Read the model definition and answer for the solid it produces. Units are mm, in the model's axes. Face numbers are marked on the shaded views. A direction names the side the tool comes from. Coordinates: 2 decimals unless noted, no trailing zeros. Write each loop counter-clockwise with the first axis right and the second up, starting at its lowest first coordinate (ties: lowest second). Pieces come first, ordered by that corner, then holes. Notation, with made-up numbers: (42.5, 87) -> (64.5, 87) arc R8 cw to (64.5, 93) -> close; hole circle Ø4 at (-22.75, 32.5). An arc over 180 degrees is marked (long way). Answer as a JSON object with one key per item and string values. Group by question number.
(1) Straight lines are drawn through the part: L1, parallel to Y at x = 2.25, z = 0; L2, parallel to X at y = -5.5, z = -2.5; L3, parallel to X at y = 5, z = 1.25. For each, find the intervals that lie inside material, in ascending order.
(2) Find section D-D (x = 22.5). Give the vertices of the cut face in (y, z), then the cut area to 3 significant figures.
(3) For a pull along Y with two mould halves and no side action, classify the marked faces 3, 4 and 5 as +Y half, -Y half, draft (parallel to the pull), parting line (faces both ways), or undercut.
(4) Find section B-B (x = 14.5). Give the vertices of the cut face in (y, z).
(5) Flat-ended cylindrical pins translate along their axes: P1, Ø0.6, axis at x = 25.5, z = -6.5, coming from the +Y side; P2, Ø7, axis at y = 3.5, z = 4.5, coming from the +X side; P3, Ø6, axis at y = 0, z = 0, coming from the -X side. Find the tip coordinate at first contact, or state that the pin passes through.
(6) Find section C-C (z = -6.25). Give the vertices of the cut face in (x, y).
(7) Find section A-A (z = 0). Give the vertices of the cut face in (x, y).
(8) Which of the six approach directions +Z, -Z, +X, -X, +Y, -Y give full straight-line access (tool end or side, diameter ignored) to the marked faces 1 and 2?
from build123d import *

# Parameters (mm, degrees)
SKETCH1_W           = 28.5
SKETCH1_H           = 15
SKETCH1_R           = 4.25
BOSS_EXTRUDE1_DEPTH = 6.2
SKETCH2_W           = 5
SKETCH2_H           = 15
BOSS_EXTRUDE2_DEPTH = 15
SKETCH3_W           = 5
SKETCH3_H           = 15
BOSS_EXTRUDE3_DEPTH = 5
CUT_EXTRUDE2_START  = 2
CUT_EXTRUDE2_DEPTH  = 1
CUT_EXTRUDE3_START  = 3
CUT_EXTRUDE3_DEPTH  = 2
FILLET1_R           = 3


with BuildPart() as part:
    # Sketch1 → Boss-Extrude1 (new body)
    with BuildSketch(Plane(origin=(0, 0, 0), x_dir=(0, 0, -1), z_dir=(1, 0, 0))):
        Rectangle(SKETCH1_W, SKETCH1_H)
        with Locations(Location((0, 0, 0), (0, 0, 180))):
            Circle(SKETCH1_R, mode=Mode.SUBTRACT)
    extrude(amount=BOSS_EXTRUDE1_DEPTH)

    # Sketch2 → Boss-Extrude2 (add)
    with BuildSketch(Plane(origin=(6.2, 0, 0), x_dir=(0, 0, -1), z_dir=(1, 0, 0))):
        with Locations((-11.75, 0)):
            Rectangle(SKETCH2_W, SKETCH2_H)
        with Locations((11.75, 0)):
            Rectangle(SKETCH2_W, SKETCH2_H)
    extrude(amount=BOSS_EXTRUDE2_DEPTH)

    # Sketch3 → Boss-Extrude3 (add)
    with BuildSketch(Plane(origin=(21.2, 0, 0), x_dir=(0, 0, -1), z_dir=(1, 0, 0))):
        with Locations((-11.75, 0)):
            Rectangle(SKETCH3_W, SKETCH3_H)
        with BuildLine():
            Line((8.525, -0.9), (8.525, 7.5))
            Line((8.525, 7.5), (-8.525, 7.5))
            Line((-8.525, 7.5), (-8.525, -0.9))
            Line((-8.525, -0.9), (-3.64039833, -0.9))
            ThreePointArc((-3.64039833, -0.9), (-0.453324532, 3.72249874), (3.75, 0))
            ThreePointArc((3.75, 0), (3.72249874, -0.453324532), (3.64039833, -0.9))
            Line((3.64039833, -0.9), (8.525, -0.9))
        make_face()
        with BuildLine():
            Line((-9.25, -7.5), (14.25, -7.5))
            Line((14.25, -7.5), (14.25, 7.5))
            Line((14.25, 7.5), (9.125, 7.5))
            Line((9.125, 7.5), (9.125, -1.5))
            Line((9.125, -1.5), (3.436931771, -1.5))
            ThreePointArc((3.436931771, -1.5), (0, -3.75), (-3.436931771, -1.5))
            Line((-3.436931771, -1.5), (-9.125, -1.5))
            Line((-9.125, -1.5), (-9.125, 7.5))
            Line((-9.125, 7.5), (-9.25, 7.5))
            Line((-9.25, 7.5), (-9.25, -7.5))
        make_face()
        with BuildLine():
            Line((-8.525, 7.5), (-9.125, 7.5))
            Line((-9.125, 7.5), (-9.125, -1.5))
            Line((-9.125, -1.5), (-3.436931771, -1.5))
            ThreePointArc((-3.436931771, -1.5), (-3.551358943, -1.204304638), (-3.64039833, -0.9))
            Line((-3.64039833, -0.9), (-8.525, -0.9))
            Line((-8.525, -0.9), (-8.525, 7.5))
        make_face()
        with BuildLine():
            Line((9.125, -1.5), (9.125, 7.5))
            Line((9.125, 7.5), (8.525, 7.5))
            Line((8.525, 7.5), (8.525, -0.9))
            Line((8.525, -0.9), (3.64039833, -0.9))
            ThreePointArc((3.64039833, -0.9), (3.551358943, -1.204304638), (3.436931771, -1.5))
            Line((3.436931771, -1.5), (9.125, -1.5))
        make_face()
    extrude(amount=BOSS_EXTRUDE3_DEPTH)

    # Sketch3<6> → Cut-Extrude2 (cut)
    with BuildSketch(Plane(origin=(21.2, 0, 0), x_dir=(0, 0, -1), z_dir=(1, 0, 0)).offset(CUT_EXTRUDE2_START)):
        with BuildLine():
            Line((8.525, -0.9), (8.525, 7.5))
            Line((8.525, 7.5), (-8.525, 7.5))
            Line((-8.525, 7.5), (-8.525, -0.9))
            Line((-8.525, -0.9), (-3.64039833, -0.9))
            ThreePointArc((-3.64039833, -0.9), (-0.453324532, 3.72249874), (3.75, 0))
            ThreePointArc((3.75, 0), (3.72249874, -0.453324532), (3.64039833, -0.9))
            Line((3.64039833, -0.9), (8.525, -0.9))
        make_face()
        with BuildLine():
            Line((-8.525, 7.5), (-9.125, 7.5))
            Line((-9.125, 7.5), (-9.125, -1.5))
            Line((-9.125, -1.5), (-3.436931771, -1.5))
            ThreePointArc((-3.436931771, -1.5), (-3.551358943, -1.204304638), (-3.64039833, -0.9))
            Line((-3.64039833, -0.9), (-8.525, -0.9))
            Line((-8.525, -0.9), (-8.525, 7.5))
        make_face()
        with BuildLine():
            Line((9.125, -1.5), (9.125, 7.5))
            Line((9.125, 7.5), (8.525, 7.5))
            Line((8.525, 7.5), (8.525, -0.9))
            Line((8.525, -0.9), (3.64039833, -0.9))
            ThreePointArc((3.64039833, -0.9), (3.551358943, -1.204304638), (3.436931771, -1.5))
            Line((3.436931771, -1.5), (9.125, -1.5))
        make_face()
    extrude(amount=CUT_EXTRUDE2_DEPTH, mode=Mode.SUBTRACT)

    # Sketch3<7> → Cut-Extrude3 (cut)
    with BuildSketch(Plane(origin=(21.2, 0, 0), x_dir=(0, 0, -1), z_dir=(1, 0, 0)).offset(CUT_EXTRUDE3_START)):
        with BuildLine():
            Line((8.525, -0.9), (8.525, 7.5))
            Line((8.525, 7.5), (-8.525, 7.5))
            Line((-8.525, 7.5), (-8.525, -0.9))
            Line((-8.525, -0.9), (-3.64039833, -0.9))
            ThreePointArc((-3.64039833, -0.9), (-0.453324532, 3.72249874), (3.75, 0))
            ThreePointArc((3.75, 0), (3.72249874, -0.453324532), (3.64039833, -0.9))
            Line((3.64039833, -0.9), (8.525, -0.9))
        make_face()
    extrude(amount=CUT_EXTRUDE3_DEPTH, mode=Mode.SUBTRACT)

    # Fillet1
    fillet1_edges = [part.edges().sort_by_distance(p)[0] for p in [
        (13.1, -7.5, -14.25),
        (13.1, -7.5, 14.25),
        (13.1, 7.5, 14.25),
        (13.1, 7.5, -14.25),
    ]]
    fillet(fillet1_edges, radius=FILLET1_R)


solid = part.part
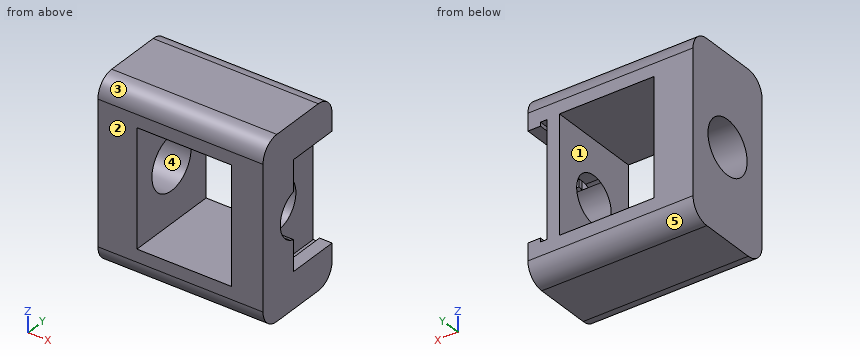
Results below:
{
 "1": {"L1": "y = -7.5 to -4.25, 4.25 to 7.5", "L2": "x = 0 to 6.2, 21.2 to 26.2", "L3": "x = 0 to 6.2, 21.2 to 23.2"},
 "2": {"outline": "(-7.5, -11.25) arc R3 ccw to (-4.5, -14.25) -> (4.5, -14.25) arc R3 ccw to (7.5, -11.25) -> (7.5, 11.25) arc R3 ccw to (4.5, 14.25) -> (-4.5, 14.25) arc R3 ccw to (-7.5, 11.25) -> close; hole circle Ø7.5 at (0, 0)", "area": "376 mm2"},
 "3": {"face 3": "-Y half", "face 4": "undercut", "face 5": "+Y half"},
 "4": {"outline": "(-7.5, -11.25) arc R3 ccw to (-4.5, -14.25) -> (4.5, -14.25) arc R3 ccw to (7.5, -11.25) -> (7.5, -9.25) -> (-7.5, -9.25) -> close; (-7.5, 9.25) -> (7.5, 9.25) -> (7.5, 11.25) arc R3 ccw to (4.5, 14.25) -> (-4.5, 14.25) arc R3 ccw to (-7.5, 11.25) -> close"},
 "5": {"P1": "stops at y = -0.9", "P2": "stops at x = 23.2", "P3": "passes through"},
 "6": {"outline": "(0, -7.5) -> (6.2, -7.5) -> (6.2, 7.5) -> (0, 7.5) -> close; (21.2, -7.5) -> (26.2, -7.5) -> (26.2, -0.9) -> (24.2, -0.9) -> (24.2, -1.5) -> (23.2, -1.5) -> (23.2, 7.5) -> (21.2, 7.5) -> close"},
 "7": {"outline": "(0, -7.5) -> (6.2, -7.5) -> (6.2, -4.25) -> (0, -4.25) -> close; (0, 4.25) -> (6.2, 4.25) -> (6.2, 7.5) -> (0, 7.5) -> close; (21.2, -7.5) -> (26.2, -7.5) -> (26.2, -3.75) -> (21.2, -3.75) -> close; (21.2, 3.75) -> (23.2, 3.75) -> (23.2, 7.5) -> (21.2, 7.5) -> close"},
 "8": {"face 1": "+Y, -Y", "face 2": "+Z, -Z, +X, -X, -Y"}
}
